from build123d import *

# Parameters (mm, degrees)
SKETCH1_R           = 2
BOSS_EXTRUDE1_DEPTH = 26.5
CUT_EXTRUDE2_START  = -1
SKETCH2_R           = 2.498108329
SKETCH2_R_2         = 1.9
CUT_EXTRUDE2_DEPTH  = 0.25
CUT_EXTRUDE3_START  = -1.25
SKETCH3_R           = 2.5
SKETCH3_R_2         = 1.9
CUT_EXTRUDE3_DEPTH  = 0.25
CHAMFER1_SIZE       = 0.25


with BuildPart() as part:
    # Sketch1 → Boss-Extrude1 (new body)
    with BuildSketch(Plane(origin=(0, 0, 0), x_dir=(0, 0, -1), z_dir=(1, 0, 0))):
        Circle(SKETCH1_R)
    extrude(amount=BOSS_EXTRUDE1_DEPTH)

    # Sketch2 → Cut-Extrude2 (cut)
    with BuildSketch(Plane(origin=(26.5, 0, 0), x_dir=(0, 0, -1), z_dir=(1, 0, 0)).offset(CUT_EXTRUDE2_START)):
        Circle(SKETCH2_R)
        Circle(SKETCH2_R_2, mode=Mode.SUBTRACT)
    extrude(amount=-CUT_EXTRUDE2_DEPTH, mode=Mode.SUBTRACT)

    # Sketch3 → Cut-Extrude3 (cut)
    with BuildSketch(Plane.ZY.offset(CUT_EXTRUDE3_START)):
        Circle(SKETCH3_R)
        with Locations(Location((0, 0, 0), (0, 0, 180))):
            Circle(SKETCH3_R_2, mode=Mode.SUBTRACT)
    extrude(amount=CUT_EXTRUDE3_DEPTH, mode=Mode.SUBTRACT)

    # Chamfer1
    chamfer1_edges = [part.edges().sort_by_distance(p)[0] for p in [
        (0, 0, 2),
        (26.5, 0, 2),
    ]]
    chamfer(chamfer1_edges, length=CHAMFER1_SIZE)


solid = part.part
Can you work these out from the model? Positions are in its coordinate system, mm. Give positions to 0.01 mm unless a question says otherwise; leave off trailing zeros. Order: outer loops, then holes, each group sorted by start corner. A loop starts at its lowest first (then second) coordinate and runs counter-clockwise, first axis right, second up. Notation, with made-up numbers: M -23.5,-10.5 L -11.5,-10.5 A9 ccw -11.5,-1.5 Z; hole C -19.75,-12.5 d8. An arc over 180 degrees is marked long. Use one line per item in the form item = value. Start each with the question number.
Item 1: If I drill on line 1 along Z through (x, y) = (4.5, -0.1); line 2 along Z through (x, y) = (5.5, -1.5); line 3 along Y through (x, z) = (9.5, -0.8), over which ranges is the centre line in solid material (lowest first)?
Item 2: If we section it at A-A (x = 8.75): Write out the boundary of the cut face in (y, z), then the cut area to 3 significant figures.
Item 3: Will this pin go through, and if not, where does the flat tip stop? pin 1 Ø1.5 at (y, z) = (-1.5, 1.5) entering from -X.
Outcome:
q1.line_1 = -2 to 2
q1.line_2 = -1.32 to 1.32
q1.line_3 = -1.83 to 1.83
q2.outline = C 0,0 d4
q2.area = 12.6 mm2
q3.pin_1 = 0
